Input: part model. Units: mm. Frame: model coordinates. Round coordinates to 2 decimals unless told otherwise and drop trailing zeros. Write each loop counter-clockwise with the first axis right and the second up, starting at its lowest first coordinate (ties: lowest second). Pieces come first, ordered by that corner, then holes. Notation, with made-up numbers: (73.25, 3) -> (108.25, 3) arc R33 ccw to (108.25, 42) -> close; hole circle Ø3 at (74, -21). An arc over 180 degrees is marked (long way). Write item = value, one per line. Start each with the question number.
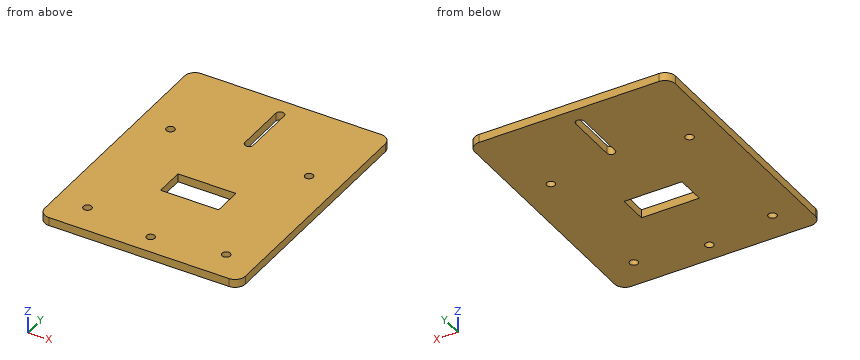
Autodesk Inventor part; units mm, degrees
ref_plane "YZ Plane" through (0, 0, 0) normal (1, 0, 0) x (0, 1, 0)
ref_plane "XZ Plane" through (0, 0, 0) normal (0, 1, 0) x (-1, 0, 0)
ref_plane "XY Plane" through (0, 0, 0) normal (0, 0, 1) x (1, 0, 0)
sketch "Эскиз1" plane through (0, 0, 0) normal (0, 0, 1) x (1, 0, 0)
  line L0 (5, 0) -> (92, 0)
  line L1 (97, 5) -> (97, 118)
  line L2 (92, 123) -> (5, 123)
  line L3 (0, 118) -> (0, 5)
  arc A0 (5, 123) -> (0, 118) centre (5, 118) ccw
  arc A1 (97, 118) -> (92, 123) centre (92, 118) ccw
  arc A2 (92, 0) -> (97, 5) centre (92, 5) ccw
  arc A3 (0, 5) -> (5, 0) centre (5, 5) ccw
  arc A4 (46.5, 89) -> (50.5, 89) centre (48.5, 89) ccw
  arc A5 (50.5, 114) -> (46.5, 114) centre (48.5, 114) ccw
  line L4 (46.5, 89) -> (46.5, 114)
  line L5 (50.5, 114) -> (50.5, 89)
  circle A6 centre (48.5, 9.5) radius 2
  line L6 (34.5, 41) -> (62.5, 41)
  line L7 (62.5, 41) -> (62.5, 55)
  line L8 (62.5, 55) -> (34.5, 55)
  line L9 (34.5, 55) -> (34.5, 41)
  circle A7 centre (15, 14.5) radius 2
  circle A8 centre (15, 81.5) radius 2
  circle A9 centre (82, 81.5) radius 2
  circle A10 centre (82, 14.5) radius 2
  point P0 (0, 0)
  point P1 (97, 123)
  point P2 (0, 123)
  dimension "d10" = 5
  dimension "d21" = 4
  dimension "d22" = 4
  dimension "d23" = 4
  dimension "d29" = 28
  dimension "d30" = 14
extrude "Выдавливание2" add sketch "Эскиз1" along normal blind 4
properties part number "Адаптер для считывателя Bolid Proxy-2MA часть 2"
1. Section A-A (y = 14.5). Output: boundary loops of the cut face in (x, z), then the cut area to 3 significant figures.
2. Line query: line 1 along Y through (x, z) = (82, 0.95); line 2 along X through (y, z) = (110, 1.5); line 3 along Y through (x, z) = (54, 0.2). Output: solid intervals per line, ascending.
3. Section C-C (y = 92.5). Output: boundary loops of the cut face in (x, z).
4. Section B-B (x = 41.5). Output: boundary loops of the cut face in (y, z).
5. Section D-D (z = 1.05). Output: boundary loops of the cut face in (x, y), then the cut area to 3 significant figures.
Check sheet entries:
q1.outline = (0, 0) -> (13, 0) -> (13, 4) -> (0, 4) -> close; (17, 0) -> (80, 0) -> (80, 4) -> (17, 4) -> close; (84, 0) -> (97, 0) -> (97, 4) -> (84, 4) -> close
q1.area = 356 mm2
q2.line_1 = 0 to 12.5, 16.5 to 79.5, 83.5 to 123
q2.line_2 = 0 to 46.5, 50.5 to 97
q2.line_3 = 0 to 41, 55 to 123
q3.outline = (0, 0) -> (46.5, 0) -> (46.5, 4) -> (0, 4) -> close; (50.5, 0) -> (97, 0) -> (97, 4) -> (50.5, 4) -> close
q4.outline = (0, 0) -> (41, 0) -> (41, 4) -> (0, 4) -> close; (55, 0) -> (123, 0) -> (123, 4) -> (55, 4) -> close
q5.outline = (0, 5) arc R5 ccw to (5, 0) -> (92, 0) arc R5 ccw to (97, 5) -> (97, 118) arc R5 ccw to (92, 123) -> (5, 123) arc R5 ccw to (0, 118) -> close; hole circle Ø4 at (15, 14.5); hole circle Ø4 at (15, 81.5); hole (34.5, 41) -> (62.5, 41) -> (62.5, 55) -> (34.5, 55) -> close; hole circle Ø4 at (48.5, 9.5); hole (46.5, 89) arc R2 ccw to (50.5, 89) -> (50.5, 114) arc R2 ccw to (46.5, 114) -> close; hole circle Ø4 at (82, 14.5); hole circle Ø4 at (82, 81.5)
q5.area = 11,300 mm2
